from build123d import *

# Parameters (mm, degrees)
BOSS_EXTRU_1_DEPTH      = 4
ESQUISSE2_W             = 1
ESQUISSE2_H             = 2
ESQUISSE2_H_2           = 2.130975397
BOSS_EXTRU_2_DEPTH      = 95
ESQUISSE3_W             = 4
ESQUISSE3_H             = 10
BOSS_EXTRU_3_DEPTH      = 4
ESQUISSE4_W             = 10
ESQUISSE4_H             = 4
BOSS_EXTRU_4_DEPTH      = 4
ESQUISSE6_W             = 5
ESQUISSE6_H             = 29.43
BOSS_EXTRU_5_DEPTH      = 4
BOSS_EXTRU_6_DEPTH      = 50
BOSS_EXTRU_6_DEPTH_BACK = 5


with BuildPart() as part:
    # Esquisse1 → Boss.-Extru.1 (new body)
    with BuildSketch(Plane.XY):
        Polygon((0.6, 0), (-0.6, 0), (-1.691910703, 3), (-2.891910703, 3), (-3.983821406, 0), (-5.183821406, 0), (-6.275732108, 3), (-7.475732108, 3), (-8.567642811, 0), (-9.767642811, 0), (-10.859553514, 3), (-12.059553514, 3), (-13.151464217, 0), (-14.351464217, 0), (-15.44337492, 3), (-16.64337492, 3), (-17.735285622, 0), (-18.935285622, 0), (-20.027196325, 3), (-21.227196325, 3), (-22.319107028, 0), (-23.519107028, 0), (-24.611017731, 3), (-25.811017731, 3), (-26.902928434, 0), (-28.102928434, 0), (-29.194839136, 3), (-30.394839136, 3), (-31.486749839, 0), (-32.686749839, 0), (-33.778660542, 3), (-34.978660542, 3), (-36.070571245, 0), (-37.270571245, 0), (-38.362481948, 3), (-39.562481948, 3), (-40.65439265, 0), (-41.85439265, 0), (-42.946303353, 3), (-44.146303353, 3), (-45.221021012, -0.00977063), (-46.4210099, -0.004606433), (-47.5, 3.000064821), (-47.5, -4), (47.5, -4), (47.5, 3.000064821), (46.438214056, 0), (45.238214056, 0), (44.146303353, 3), (42.946303353, 3), (41.85439265, 0), (40.65439265, 0), (39.562481948, 3), (38.362481948, 3), (37.270571245, 0), (36.070571245, 0), (34.978660542, 3), (33.778660542, 3), (32.686749839, 0), (31.486749839, 0), (30.394839136, 3), (29.194839136, 3), (28.102928434, 0), (26.902928434, 0), (25.811017731, 3), (24.611017731, 3), (23.519107028, 0), (22.319107028, 0), (21.227196325, 3), (20.027196325, 3), (18.935285622, 0), (17.735285622, 0), (16.64337492, 3), (15.44337492, 3), (14.351464217, 0), (13.151464217, 0), (12.059553514, 3), (10.859553514, 3), (9.767642811, 0), (8.567642811, 0), (7.475732108, 3), (6.275732108, 3), (5.183821406, 0), (3.983821406, 0), (2.891910703, 3), (1.691910703, 3), align=None)
    extrude(amount=-BOSS_EXTRU_1_DEPTH)

    # Esquisse2 → Boss.-Extru.2 (add)
    with BuildSketch(Plane.ZY.offset(47.5)):
        with Locations((-4.5, -3)):
            Rectangle(ESQUISSE2_W, ESQUISSE2_H)
        with Locations((0.5, -2.934512301)):
            Rectangle(ESQUISSE2_W, ESQUISSE2_H_2)
    extrude(amount=-BOSS_EXTRU_2_DEPTH)

    # Esquisse3 → Boss.-Extru.3 (add)
    with BuildSketch(Plane(origin=(0, 0, -4), x_dir=(-1, 0, 0), z_dir=(0, 0, -1))):
        with Locations((49.5, 3)):
            Rectangle(ESQUISSE3_W, ESQUISSE3_H)
    extrude(amount=-BOSS_EXTRU_3_DEPTH)

    # Esquisse4 → Boss.-Extru.4 (add)
    with BuildSketch(Plane.ZY.offset(51.5)):
        with Locations((-9, 6)):
            Rectangle(ESQUISSE4_W, ESQUISSE4_H)
    extrude(amount=-BOSS_EXTRU_4_DEPTH)

    # Esquisse6 → Boss.-Extru.5 (add)
    with BuildSketch(Plane.ZY.offset(51.5)):
        with Locations((-11.5, 18.715)):
            Rectangle(ESQUISSE6_W, ESQUISSE6_H)
    extrude(amount=-BOSS_EXTRU_5_DEPTH)

    # Esquisse7 → Boss.-Extru.6 (add, two sides: drawn at the far end of the back side and taken through both)
    with BuildSketch(Plane(origin=(0, 0, -14), x_dir=(-1, 0, 0), z_dir=(0, 0, -1)).offset(-BOSS_EXTRU_6_DEPTH_BACK)):
        Polygon((47.543968479, 63.053350001), (47.543968479, 23.053350001), (51.550036892, 28.053350001), (52.543968479, 28.423350001), (52.543968479, 43.303350001), (51.550036892, 45.973350001), (51.550036892, 55.49434682), align=None)
    extrude(amount=BOSS_EXTRU_6_DEPTH + BOSS_EXTRU_6_DEPTH_BACK)


solid = part.part
Work out the finished part from the listing and answer in its coordinate system (mm). A direction names the side the tool comes from. Round coordinates to 2 decimals unless told otherwise and drop trailing zeros. Write each loop counter-clockwise with the first axis right and the second up, starting at its lowest first coordinate (ties: lowest second). Pieces come first, ordered by that corner, then holes. Notation, with made-up numbers: (-28.5, -24.5) - (21.5, -24.5) arc R20 cw to (21.5, -4.5) - close; hole circle Ø9 at (11.25, 68). An arc over 180 degrees is marked (long way). Answer in a Markdown table with one row per item. Add a question column.
1. For faces 1 (the flat face through (-44.676, 1.516, -1.972)), 2 (the flat face through (-49, -2, -2)), 3 (the flat face through (-50, 4, -9)), determine the directions among +Z, -Z, +X, -X, +Y, -Y from which every point of the face is accessible in a straight line to the end or side of a thin tool.
2. A cutting plane is placed at C-C, the plane y = 1.5. Count the separate pieces of the cut face and the enclosed holes in it, and give its area (3 significant figures).
3. A cutting plane is placed at D-D, the plane y = 53. Determine the outline of the cut face in (x, z), and give its area (3 significant figures).
4. Given pin 1 (1.5 mm diameter, centred on y = 15.5, z = -15.5, fed in from +X); pin 2 (5 mm diameter, centred on y = 21.5, z = -31, fed in from -X); pin 3 (1 mm diameter, centred on x = -34, z = -1, fed in from +Y); pin 4 (12 mm diameter, centred on y = 16, z = -18, fed in from +X), each flat-ended and moving along its own axis, determine where each tip first touches the part or whether it passes through.
5. Find the intervals of material crossed by line 1 along X through (y, z) = (55.5, -48); line 2 along X through (y, z) = (35, -48); line 3 along Y through (x, z) = (2.5, -2), in increasing order. Write a range as from..to.
6. A cutting plane is placed at B-B, the plane y = 31. Determine the outline of the cut face in (x, z), and give its area (3 significant figures).
7. A cutting plane is placed at A-A, the plane z = -50.5. Determine the outline of the cut face in (x, y).
Worked out:
| question | item | result |
|---|---|---|
| 1 | face 1 | +Z, -Z, +Y |
| 1 | face 2 | +Z, -Z, -X, -Y |
| 1 | face 3 | -Z, +X, -X, -Y |
| 2 | separate pieces | 22 |
| 2 | enclosed holes | 0 |
| 2 | area | 204 mm^2 |
| 3 | outline | (-51.55, -64) - (-47.54, -64) - (-47.54, -9) - (-51.55, -9) - close |
| 3 | area | 220 mm^2 |
| 4 | pin 1 | through |
| 4 | pin 2 | x = -48.3 |
| 4 | pin 3 | y = 3 |
| 4 | pin 4 | x = -47.5 |
| 5 | line 1 | -51.55..-47.54 |
| 5 | line 2 | -52.54..-47.54 |
| 5 | line 3 | -4..3 |
| 6 | outline | (-52.54, -64) - (-47.54, -64) - (-47.54, -14) - (-47.5, -14) - (-47.5, -9) - (-52.54, -9) - close |
| 6 | area | 275 mm^2 |
| 7 | outline | (-52.54, 28.42) - (-51.55, 28.05) - (-47.54, 23.05) - (-47.54, 63.05) - (-51.55, 55.49) - (-51.55, 45.97) - (-52.54, 43.3) - close |
